Check sheet for the modelled part. Datum: model origin and axes. Units: mm. A direction names the side the tool comes from. Round coordinates to 2 decimals unless told otherwise and drop trailing zeros. Write each loop counter-clockwise with the first axis right and the second up, starting at its lowest first coordinate (ties: lowest second). Pieces come first, ordered by that corner, then holes. Notation, with made-up numbers: (-6, 35) -> (22, 35) arc R25 ccw to (22, 59) -> close; hole circle Ø4 at (81, 85). An arc over 180 degrees is marked (long way). Write item = value, one per line.
from build123d import *

# Parameters (mm, degrees)
F0_W     = 19.05
F0_H     = 19.05
F1_DEPTH = 50.8
F2_W     = 4.3630654678
F2_H     = 20.508804819
F3_DEPTH = 25.4
F4_W     = 4.3975393042
F4_H     = 20.508804819
F5_DEPTH = 25.4
F6_W     = 4.3544375803
F6_H     = 20.508804819
F7_DEPTH = 6.35
F8_W     = 6.35
F8_H     = 4.6250596642
F9_DEPTH = 25.4


# Not quite as in the source:
# - a feature names something its author has since deleted; it is built from what else it names


with BuildPart() as f1:
    # F0 (on Top) → F1 (new body)
    with BuildSketch(Plane.XY):
        Rectangle(F0_W, F0_H)
    extrude(amount=F1_DEPTH)

    # F2 (on face) → F3 (cut)
    with BuildSketch(Plane.YZ.offset(9.525)):
        with Locations((7.3434672661, 40.5455975905)):
            Rectangle(F2_W, F2_H)
    extrude(amount=-F3_DEPTH, mode=Mode.SUBTRACT)

    # F4 (on face) → F5 (cut)
    with BuildSketch(Plane(origin=(0, 5.1619345322, 0), x_dir=(-1, 0, 0), z_dir=(0, 1, 0))):
        with Locations((7.3262303479, 40.5455975905)):
            Rectangle(F4_W, F4_H)
    extrude(amount=-F5_DEPTH, mode=Mode.SUBTRACT)

    # F6 (on face) → F7 (cut)
    with BuildSketch(Plane(origin=(-5.1274606958, 0, 0), x_dir=(0, -1, 0), z_dir=(-1, 0, 0))):
        with Locations((-2.9847157421, 40.5455975905)):
            Rectangle(F6_W, F6_H)
    extrude(amount=-F7_DEPTH, mode=Mode.SUBTRACT)

    # F8 (on face) → F9 (cut)
    with BuildSketch(Plane(origin=(0, 0.8074969519, 0), x_dir=(-1, 0, 0), z_dir=(0, 1, 0))):
        with Locations((1.9524606958, 38.9165244997)):
            Rectangle(F8_W, F8_H)
    extrude(amount=-F9_DEPTH, mode=Mode.SUBTRACT)


solid = f1.part
(1) Sectioned sample at A-A on x = -1. Enter the section's corners in (y, z) (1 decimal).
Worked answers:
outline = (-9.5, 0) -> (9.5, 0) -> (9.5, 30.3) -> (0.8, 30.3) -> (0.8, 36.6) -> (-9.5, 36.6) -> close; (-9.5, 41.2) -> (0.8, 41.2) -> (0.8, 50.8) -> (-9.5, 50.8) -> close
(2) Go/stop test with flat-tipped pins: P1, Ø1, axis at x = 0, z = 42, coming from the +Y side; P2, Ø3, axis at y = -6, z = 44, coming from the -X side; P3, Ø4, axis at x = 6, z = 35.5, coming from the +Y side. Record where each tip stops, or that it passes through.
Worked answers:
P1 = 0.81
P2 = -5.13
P3 = 5.16
(3) Release check for a two-part mould opening along Z. For faces 1 (the flat face through (5, 5.162, 40)), 2 (the flat face through (0, 0, 0)), 3 (the flat face through (1.223, 1, 40)) record: pulls with the +Z half, pulls with the -Z half, needs draft (parallel to the pull), parting line crosses it, or undercut.
Worked answers:
face_1 = needs draft
face_2 = pulls with the -Z half
face_3 = undercut
(4) Access from +Z, -Z, +X, -X, +Y, -Y to the whole of each face (thin tool, end or side, straight path). Record for faces 4 (the flat face through (-2, -4, 36.604)), 5 (the flat face through (0, 9.525, 15)), 6 (the flat face through (-5.127, -4, 33)), 7 (the flat face through (-2, 0.807, 46)).
Worked answers:
face_4 = -X, +Y, -Y
face_5 = +Z, -Z, +X, -X, +Y
face_6 = +Z, -X, +Y, -Y
face_7 = +Z, -X, +Y
(5) Material ranges on L1, parallel to Z at x = -2, y = -0.5; L2, parallel to Z at x = 0.75, y = 6; L3, parallel to X at y = -0.5, z = 44.5 (3 decimals), recorded low to high. Write a range as [from, to].
Worked answers:
L1 = [0, 36.6], [41.23, 50.8]
L2 = [0, 30.29]
L3 = [-5.127, 9.525]
(6) Sectioned sample at B-B on y = -6. Enter the section's corners in (x, z) (3 decimals), then the cut area to 3 significant figures.
Worked answers:
outline = (-9.525, 0) -> (9.525, 0) -> (9.525, 50.8) -> (-5.127, 50.8) -> (-5.127, 41.229) -> (1.223, 41.229) -> (1.223, 36.604) -> (-5.127, 36.604) -> (-5.127, 30.291) -> (-9.525, 30.291) -> close
area = 848 mm²
(7) Sectioned sample at C-C on z = 45. Enter the section's corners in (x, y) (1 decimal), then the cut area to 3 significant figures.
Worked answers:
outline = (-5.1, -9.5) -> (9.5, -9.5) -> (9.5, 5.2) -> (1.2, 5.2) -> (1.2, 0.8) -> (-5.1, 0.8) -> close
area = 188 mm²
(8) Sectioned sample at D-D on x = 8. Enter the section's corners in (y, z) (3 decimals).
Worked answers:
outline = (-9.525, 0) -> (9.525, 0) -> (9.525, 30.291) -> (5.162, 30.291) -> (5.162, 50.8) -> (-9.525, 50.8) -> close
